from build123d import *

# Parameters (mm, degrees)
SKETCH1_W                                       = 50
SKETCH1_H                                       = 38
BOSS_EXTRUDE1_DEPTH                             = 10
M10X1_5_TAPPED_HOLE1_D                          = 8.5
CBORE_FOR_M5_SOCKET_HEAD_CAP_SCREW1_D           = 5.5
CBORE_FOR_M5_SOCKET_HEAD_CAP_SCREW1_CBORE_D     = 9.5
CBORE_FOR_M5_SOCKET_HEAD_CAP_SCREW1_CBORE_DEPTH = 5.4


with BuildPart() as part:
    # Sketch1 → Boss-Extrude1 (new body)
    with BuildSketch(Plane(origin=(0, 0, 0), x_dir=(0, 0, -1), z_dir=(1, 0, 0))):
        with Locations((0, 19)):
            Rectangle(SKETCH1_W, SKETCH1_H)
    extrude(amount=BOSS_EXTRUDE1_DEPTH)

    # M10x1.5 Tapped Hole1 (through all)
    with Locations(Plane(origin=(10, 0, 0), x_dir=(0, 0, -1), z_dir=(1, 0, 0))):
        with Locations((0, 25)):
            Hole(M10X1_5_TAPPED_HOLE1_D / 2)

    # CBORE for M5 Socket Head Cap Screw1 (through all)
    with Locations(Plane(origin=(10, 0, 0), x_dir=(0, 0, -1), z_dir=(1, 0, 0))):
        with Locations((18, 6), (-18, 6)):
            CounterBoreHole(CBORE_FOR_M5_SOCKET_HEAD_CAP_SCREW1_D / 2, CBORE_FOR_M5_SOCKET_HEAD_CAP_SCREW1_CBORE_D / 2, CBORE_FOR_M5_SOCKET_HEAD_CAP_SCREW1_CBORE_DEPTH)


solid = part.part
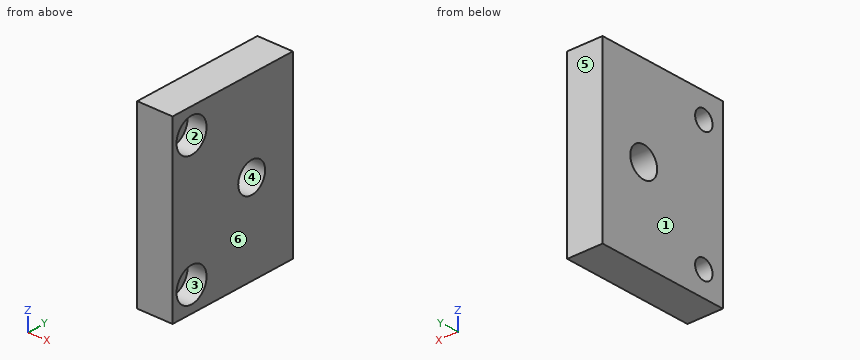
Design review of the part built by this model. Coordinates are the model's own, in mm. Face numbers are marked on the shaded views. A direction names the side the tool comes from. Give positions to 0.01 mm unless a question says otherwise; leave off trailing zeros. Write each loop counter-clockwise with the first axis right and the second up, starting at its lowest first coordinate (ties: lowest second). Pieces come first, ordered by that corner, then holes. Notation, with made-up numbers: M -15.5,-24 L 9.5,-24 A15 cw 9.5,3 Z; hole C 20,25.25 d4. An arc over 180 degrees is marked long. Answer as a JSON object with one key per item and string values. Group by question number.
1) Tool access review of the marked faces 1 and 2: name each direction out of +Z, -Z, +X, -X, +Y, -Y from which nothing blocks a thin tool from reaching the whole face with its end or side.
2) We need section C-C (x = 6.5). Give the boundary of the cut face in (y, z).
3) Mouldability with a two-part tool opening along Y and no side actions: class the marked faces 3, 4, 5 and 6 as released by +Y, released by -Y, zero draft, split by the parting line, or undercut.
4) For line 1 along Y through (x, z) = (3.25, 0); line 2 along Y through (x, z) = (7.1, -18); line 3 along Z through (x, y) = (2.25, 7.5), list the stretches that pass through material, from the lowest coordinate up.
5) Clearance check with flat-ended pins moving along their axes: pin 1 Ø1 at (x, z) = (8, 6) entering from -Y; pin 2 Ø7 at (y, z) = (6, -18) entering from +X. State where each tip first meets the part, or that it passes through.
6) We need section A-A (z = -18). Give the boundary of the cut face in (x, y), and give its area (3 significant figures).
7) We need section B-B (y = 25). Give the boundary of the cut face in (x, z), and give its area (3 significant figures).
8) We need section D-D (y = 6). Give the boundary of the cut face in (x, z), and give its area (3 significant figures).
Answer key:
{
 "1": {"face 1": "+Z, -Z, -X, +Y, -Y", "face 2": "+X"},
 "2": {"outline": "M 0,-25 L 38,-25 L 38,25 L 0,25 Z; hole C 6,-18 d9.5; hole C 6,18 d9.5; hole C 25,0 d8.5"},
 "3": {"face 3": "undercut", "face 4": "undercut", "face 5": "released by +Y", "face 6": "zero draft"},
 "4": {"line 1": "y = 0 to 20.75, 29.25 to 38", "line 2": "y = 0 to 1.25, 10.75 to 38", "line 3": "z = -25 to -20.3, -15.7 to 15.7, 20.3 to 25"},
 "5": {"pin 1": "stops at y = 0", "pin 2": "stops at x = 4.6"},
 "6": {"outline": "M 0,0 L 10,0 L 10,1.25 L 4.6,1.25 L 4.6,3.25 L 0,3.25 Z; M 0,8.75 L 4.6,8.75 L 4.6,10.75 L 10,10.75 L 10,38 L 0,38 Z", "area": "303 mm²"},
 "7": {"outline": "M 0,-25 L 10,-25 L 10,-4.25 L 0,-4.25 Z; M 0,4.25 L 10,4.25 L 10,25 L 0,25 Z", "area": "415 mm²"},
 "8": {"outline": "M 0,-25 L 10,-25 L 10,-22.75 L 4.6,-22.75 L 4.6,-20.75 L 0,-20.75 Z; M 0,-15.25 L 4.6,-15.25 L 4.6,-13.25 L 10,-13.25 L 10,13.25 L 4.6,13.25 L 4.6,15.25 L 0,15.25 Z; M 0,20.75 L 4.6,20.75 L 4.6,22.75 L 10,22.75 L 10,25 L 0,25 Z", "area": "347 mm²"}
}
